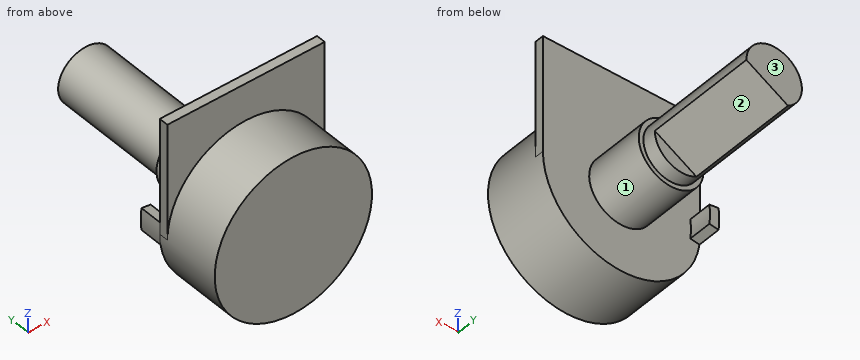
from build123d import *

# Parameters (mm, degrees)
SKETCH_1_R          = 8.5
EXTRUDE_1_DEPTH     = 7.2
EXTRUDE_2_DEPTH     = 2.5
SKETCH_3_R          = 3.5
EXTRUDE_3_DEPTH     = 6.5
SKETCH_4_R          = 3
EXTRUDE_4_DEPTH     = 13.5
CUT_EXTRUDE_START   = -12
CUT_EXTRUDE_1_DEPTH = 12
SKETCH_6_W          = 17
SKETCH_6_H          = 12.5
EXTRUDE_5_DEPTH     = 1


with BuildPart() as part:
    # 草图1 → 凸台-拉伸1 (new body)
    with BuildSketch(Plane(origin=(0, 0, 0), x_dir=(1, 0, 0), z_dir=(0, 1, 0))):
        with Locations(Location((0, 0, 0), (0, 0, 270))):
            Circle(SKETCH_1_R)
    extrude(amount=EXTRUDE_1_DEPTH)

    # 草图2 → 凸台-拉伸2 (add)
    with BuildSketch(Plane(origin=(0, 7.2, 0), x_dir=(1, 0, 0), z_dir=(0, 1, 0))):
        with BuildLine():
            Line((-7.427010516, 1.043798257), (-8.417278584, 1.182971358))
            ThreePointArc((-8.417278584, 1.182971358), (-8.5, 0), (-8.417278584, -1.182971358))
            Line((-8.417278584, -1.182971358), (-7.427010516, -1.043798257))
            ThreePointArc((-7.427010516, -1.043798257), (-7.5, 0), (-7.427010516, 1.043798257))
        make_face()
    extrude(amount=EXTRUDE_2_DEPTH)

    # 草图3 → 凸台-拉伸3 (add)
    with BuildSketch(Plane(origin=(0, 7.2, 0), x_dir=(1, 0, 0), z_dir=(0, 1, 0))):
        with Locations(Location((0, 0, 0), (0, 0, 90))):
            Circle(SKETCH_3_R)
    extrude(amount=EXTRUDE_3_DEPTH)

    # 草图4 → 凸台-拉伸4 (add)
    with BuildSketch(Plane(origin=(0, 13.7, 0), x_dir=(1, 0, 0), z_dir=(0, 1, 0))):
        with Locations(Location((0, 0, 0), (0, 0, 270))):
            Circle(SKETCH_4_R)
    extrude(amount=EXTRUDE_4_DEPTH)

    # 草图5 → 切除-拉伸1 (cut)
    with BuildSketch(Plane(origin=(0, 27.2, 0), x_dir=(1, 0, 0), z_dir=(0, 1, 0)).offset(CUT_EXTRUDE_START)):
        with BuildLine():
            Line((-1.5, 2.598076211), (3, 0))
            ThreePointArc((3, 0), (1.5, 2.598076211), (-1.5, 2.598076211))
        make_face()
    extrude(amount=CUT_EXTRUDE_1_DEPTH, mode=Mode.SUBTRACT)

    # 草图6 → 凸台-拉伸5 (add)
    with BuildSketch(Plane(origin=(0, 7.2, 0), x_dir=(1, 0, 0), z_dir=(0, 1, 0))):
        with Locations((0, -6.25)):
            Rectangle(SKETCH_6_W, SKETCH_6_H)
    extrude(amount=-EXTRUDE_5_DEPTH)


solid = part.part
Build history of the part. All positions in model axes, mm. Face numbers are marked on the shaded views. A direction names the side the tool comes from. Give positions to 0.01 mm unless a question says otherwise; leave off trailing zeros. Loops run counter-clockwise (first coordinate to the right, second up) from the corner with the lowest first, then second, coordinate; pieces in that order, holes last. Notation, with made-up numbers: (55.25, 22) - (62.25, 22) arc R25 cw to (62.25, 55) - close; hole circle Ø11 at (82, 79.5). An arc over 180 degrees is marked (long way). Write item = value, one per line. Start each with the question number.
1) Band-saw the part on A-A on z = 7.5. Give the cut face in (x, y), plus the area to 3 significant figures.
2) Probe probe 1 along Y at (x, z) = (5, -4.5); probe 2 along Y at (x, z) = (-4, 8.75); probe 3 along X at (y, z) = (2.25, 0.25). List the from-to ranges inside material, lowest first. Write a range as from..to.
3) Band-saw the part on C-C on y = 11.5. Give the cut face in (x, z), plus the area to 3 significant figures.
4) Tool access for the marked faces 1, 2 and 3: list every direction of +Z, -Z, +X, -X, +Y, -Y with a clear straight run to the whole face (end or side of a thin tool).
5) Drop flat-ended pins along their axis: pin 1 Ø8 at (x, y) = (-1, 23.5) entering from -Z; pin 2 Ø3 at (x, y) = (6, 7) entering from -Z; pin 3 Ø1 at (y, z) = (5.5, -2.5) entering from +X. Give the stop position or say it passes through.
6) Band-saw the part on D-D on z = 1.75. Give the cut face in (x, y).
7) Band-saw the part on B-B on x = 0. Give the cut face in (y, z).
Final values:
q1.outline = (-8.5, 6.2) - (-4, 6.2) - (-4, 0) - (4, 0) - (4, 6.2) - (8.5, 6.2) - (8.5, 7.2) - (-8.5, 7.2) - close
q1.area = 66.6 mm²
q2.probe_1 = 0..7.2
q2.probe_2 = 6.2..7.2
q2.probe_3 = -8.5..8.5
q3.outline = circle Ø7 at (0, 0)
q3.area = 38.5 mm²
q4.face_1 = +Y
q4.face_2 = -Z, +X, +Y
q4.face_3 = +Z, -Z, +X, -X, +Y
q5.pin_1 = -2.6
q5.pin_2 = -7.21
q5.pin_3 = 8.26
q6.outline = (-8.5, 6.2) - (-8.32, 6.2) - (-8.32, 0) - (8.32, 0) - (8.32, 6.2) - (8.5, 6.2) - (8.5, 7.2) - (3.03, 7.2) - (3.03, 13.7) - (2.44, 13.7) - (2.44, 27.2) - (-2.44, 27.2) - (-2.44, 13.7) - (-3.03, 13.7) - (-3.03, 7.2) - (-8.5, 7.2) - close
q7.outline = (0, -8.5) - (7.2, -8.5) - (7.2, -3.5) - (13.7, -3.5) - (13.7, -3) - (15.2, -3) - (15.2, -1.73) - (27.2, -1.73) - (27.2, 3) - (13.7, 3) - (13.7, 3.5) - (7.2, 3.5) - (7.2, 12.5) - (6.2, 12.5) - (6.2, 8.5) - (0, 8.5) - close
